from build123d import *

# Parameters (mm, degrees)
SKETCH_1_R          = 1.5
EXTRUDE_1_DEPTH     = 15
SKETCH_2_W          = 21.498069498
SKETCH_2_H          = 12
CUT_EXTRUDE_1_DEPTH = 50
SKETCH_3_W          = 12
SKETCH_3_H          = 16
CUT_EXTRUDE_2_DEPTH = 50
SKETCH_4_R          = 1.5
CUT_EXTRUDE_3_DEPTH = 50


with BuildPart() as part:
    # Эскиз1 → Вытянуть1 (new body)
    with BuildSketch(Plane.XY):
        with BuildLine():
            Line((1.187295832, 4.528019462), (30.355876768, 17.5))
            Line((30.355876768, 17.5), (34.911631679, 17.5))
            Line((34.911631679, 17.5), (40, 2.498964042))
            Line((40, 2.498964042), (36.034968506, 0))
            Line((36.034968506, 0), (0, 0))
            Line((0, 0), (0, 2.700586308))
            ThreePointArc((0, 2.700586308), (0.322888147, 3.790217361), (1.187295832, 4.528019462))
        make_face()
        with Locations((35.266995766, 4)):
            Circle(SKETCH_1_R, mode=Mode.SUBTRACT)
        with Locations((31.42446315, 13.771639734)):
            Circle(SKETCH_1_R, mode=Mode.SUBTRACT)
    extrude(amount=EXTRUDE_1_DEPTH)

    # Эскиз2 → Вырез-Вытянуть1 (cut)
    with BuildSketch(Plane.XZ):
        with Locations((35.749034749, 7.5)):
            Rectangle(SKETCH_2_W, SKETCH_2_H)
    extrude(amount=-CUT_EXTRUDE_1_DEPTH, mode=Mode.SUBTRACT)

    # Эскиз3 → Вырез-Вытянуть2 (cut)
    with BuildSketch(Plane(origin=(25, 0, 0), x_dir=(0, 0, -1), z_dir=(1, 0, 0))):
        with Locations((-7.5, 9.5)):
            Rectangle(SKETCH_3_W, SKETCH_3_H)
    extrude(amount=-CUT_EXTRUDE_2_DEPTH, mode=Mode.SUBTRACT)

    # Эскиз4 → Вырез-Вытянуть3 (cut)
    with BuildSketch(Plane.XZ):
        with Locations(Location((8, 7.5, 0), (0, 0, 270))):
            Circle(SKETCH_4_R)
        with Locations(Location((20, 7.5, 0), (0, 0, 270))):
            Circle(SKETCH_4_R)
    extrude(amount=-CUT_EXTRUDE_3_DEPTH, mode=Mode.SUBTRACT)


solid = part.part
The listing builds one solid part. Answer for the finished solid, in the listing's coordinates (mm). A direction names the side the tool comes from. Coordinates: 2 decimals unless noted, no trailing zeros. Write each loop counter-clockwise with the first axis right and the second up, starting at its lowest first coordinate (ties: lowest second). Pieces come first, ordered by that corner, then holes. Notation, with made-up numbers: M 52,36.5 L 82,36.5 A12 cw 82,42.5 Z; hole C 72.25,-6 d6. An arc over 180 degrees is marked long. Write each question's results on one line, items separated by ' | '.
Item 1: The part is cut by section D-D on x = 10. Determine the outline of the cut face in (y, z), and give its area (3 significant figures).
Answer below:
outline: M 0,0 L 8.45,0 L 8.45,1.5 L 1.5,1.5 L 1.5,13.5 L 8.45,13.5 L 8.45,15 L 0,15 Z | area: 43.3 mm2
Item 2: The part is cut by section B-B on x = 20. Determine the outline of the cut face in (y, z), and give its area (3 significant figures).
Answer below:
outline: M 0,0 L 12.89,0 L 12.89,1.5 L 1.5,1.5 L 1.5,6 L 0,6 Z; M 0,9 L 1.5,9 L 1.5,13.5 L 12.89,13.5 L 12.89,15 L 0,15 Z | area: 52.2 mm2
Item 3: Which of the six approach directions +Z, -Z, +X, -X, +Y, -Y give full straight-line access (tool end or side, diameter ignored) to faces 4 (the face through (37.42, 10.1, 14.24)), 5 (the face through (25, 1, 7))?
Answer below:
face 4: +Z, -Z, +X, +Y | face 5: +X, +Y, -Y
Item 4: Consider probe 1 along Z at (x, y) = (11.5, 6.25); probe 2 along Y at (x, z) = (11, 5.5); probe 3 along X at (y, z) = (4, 14.1). Determine where each line is inside the solid, lowest interval first. Write a range as [from, to].
Answer below:
probe 1: [0, 1.5], [13.5, 15] | probe 2: [0, 1.5] | probe 3: [0.48, 33.77], [36.77, 39.49]
Item 5: Given P1, Ø2.5, axis at x = 31.42, y = 13.77, coming from the -Z side; P2, Ø3.5, axis at x = 15.5, z = 9.5, coming from the +Y side; P3, Ø0.8, axis at y = 1, z = 8.5, coming from the +X side, each flat-ended and moving along its own axis, determine where each tip first touches the part or whether it passes through.
Answer below:
P1: through | P2: y = 1.5 | P3: x = 25
Item 6: The part is cut by section C-C on y = 7.5. Determine the outline of the cut face in (x, z), and give its area (3 significant figures).
Answer below:
outline: M 7.87,0 L 38.3,0 L 38.3,1.5 L 7.87,1.5 Z; M 7.87,13.5 L 38.3,13.5 L 38.3,15 L 7.87,15 Z | area: 91.3 mm2
Item 7: For a pull along X with two mould halves and no side action, classify faces 1 (the face through (34.077, 3.087, 0.74)), 2 (the face through (13, 1.5, 8)), 3 (the face through (15.567, 10.923, 0.74)) as released by +X, released by -X, zero draft, split by the parting line, or undercut.
Answer below:
face 1: undercut | face 2: zero draft | face 3: released by -X
Item 8: The part is cut by section A-A on z = 7.5. Determine the outline of the cut face in (x, y).
Answer below:
outline: M 0,0 L 6.5,0 L 6.5,1.5 L 0,1.5 Z; M 9.5,0 L 18.5,0 L 18.5,1.5 L 9.5,1.5 Z; M 21.5,0 L 25,0 L 25,1.5 L 21.5,1.5 Z
